Build history of the part. All positions in model axes, mm. Round coordinates to 2 decimals unless told otherwise and drop trailing zeros. Loops run counter-clockwise (first coordinate to the right, second up) from the corner with the lowest first, then second, coordinate; pieces in that order, holes last. Notation, with made-up numbers: (-18.5, 34) -> (-12.5, 34) arc R32 ccw to (-12.5, 64) -> close; hole circle Ø5 at (-18.5, 5.5). An arc over 180 degrees is marked (long way). Put each result on its own line as item: value. Start each with the question number.
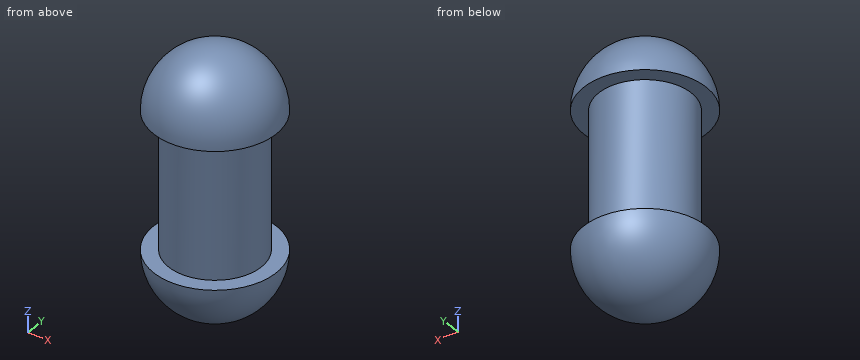
```python
from build123d import *

# Parameters (mm, degrees)
SKETCH1_R           = 15.5
BOSS_EXTRUDE1_DEPTH = 22.75


with BuildPart() as part:
    # Sketch1 → Boss-Extrude1 (new, symmetric)
    with BuildSketch(Plane.XY):
        Circle(SKETCH1_R)
    extrude(amount=BOSS_EXTRUDE1_DEPTH, both=True)

    # Sketch2 → Revolve1 (revolve)
    with BuildSketch(Plane(origin=(0, 0, 0), x_dir=(0, 0, -1), z_dir=(1, 0, 0))):
        with BuildLine():
            Line((-43.25, 0), (-22.75, 0))
            Line((-22.75, 0), (-22.75, 20.5))
            ThreePointArc((-22.75, 20.5), (-37.245689014, 14.495689014), (-43.25, 0))
        make_face()
    revolve(axis=Axis((0, 0, 0), (0, 0, 1)))

    # Mirror1: part across plane


with BuildPart() as part_1:
    add(part.part)
    add(part.part.mirror(Plane.XY))


solid = part_1.part
```
Item 1: Cut at A-A on y = 0. Write the cut outline in (x, z).
Item 2: Drop flat-ended pins along their axis: pin 1 (4 mm diameter, centred on x = -7.5, y = 14.5, fed in from +Z); pin 2 (6 mm diameter, centred on y = -6.5, z = -9.5, fed in from +X); pin 3 (1 mm diameter, centred on x = 9, y = -1, fed in from +Z). Give the stop position or say it passes through.
Item 3: Cut at D-D on x = 4.5. Write the cut outline in (y, z), then the cut area to 3 significant figures.
Item 4: Wall check: line 1 (Z direction, x = 14, y = 7); line 2 (Y direction, x = 0, z = 0); line 3 (Z direction, x = 16, y = 3). Give the ranges that are in metal, low to high. Write a range as from..to.
Item 5: Cut at C-C on z = 14. Write the cut outline in (x, y), then the cut area to 3 significant figures.
Ans:
1. outline: (-20.5, -22.75) arc R20.5 ccw to (20.5, -22.75) -> (15.5, -22.75) -> (15.5, 22.75) -> (20.5, 22.75) arc R20.5 ccw to (-20.5, 22.75) -> (-15.5, 22.75) -> (-15.5, -22.75) -> close
2. pin 1: stops at z = 37.41
2. pin 2: stops at x = 15.1
2. pin 3: stops at z = 41.38
3. outline: (-20, -22.75) arc R20 ccw to (20, -22.75) -> (14.83, -22.75) -> (14.83, 22.75) -> (20, 22.75) arc R20 ccw to (-20, 22.75) -> (-14.83, 22.75) -> (-14.83, -22.75) -> close
3. area: 2,610 mm2
4. line 1: z = -35.99..-22.75, 22.75..35.99
4. line 2: y = -15.5..15.5
4. line 3: z = -35.21..-22.75, 22.75..35.21
5. outline: circle Ø31 at (0, 0)
5. area: 755 mm2
